Geometry: final body of the model. Coordinates: model frame, mm. A direction names the side the tool comes from. Give positions to 0.01 mm unless a question says otherwise; leave off trailing zeros. Write each loop counter-clockwise with the first axis right and the second up, starting at its lowest first coordinate (ties: lowest second). Pieces come first, ordered by that corner, then holes. Notation, with made-up numbers: (-39, 57.5) - (-21, 57.5) arc R8 ccw to (-21, 67.5) - close; hole circle Ø4 at (20, -12.75). An arc over 180 degrees is marked (long way). Use CSV: the item, a comma, the result in double quotes. Start each with the question number.
(1) Section D-D on z = 5. Output: boundary loops of the cut face in (x, y), and give its area (3 significant figures).
(2) Section C-C on z = 0. Output: boundary loops of the cut face in (x, y), and give its area (3 significant figures).
(3) Line query: probe 1 along Z at (x, y) = (0, -0.5); probe 2 along Y at (x, z) = (-4, -2.25); probe 3 along Z at (x, y) = (18.5, 1.5). Output: solid intervals per line, ascending. Write a range as [from, to].
(4) Draft query along Y for faces 6 (the flat face through (4, -6.5, 2)), 7 (the flat face through (25, 0, 4)), 8 (the flat face through (4, 6.5, 2)), 9 (the flat face through (0.5, -0.1, 7.5)). Return one class per face: released by +Y, released by -Y, zero draft, split by the parting line, or undercut.
(5) Reachability of faces 1 (the flat face through (1, 0, 8)), 2 (the flat face through (19, 0, 3)), 3 (the flat face through (5, 5, 3)), 4 (the flat face through (14, 0, 7.5)), 5 (the cylindrical face through (-6.99, -0.09, -5.67)) from +Z, -Z, +X, -X, +Y, -Y: full face, straight path, thin tool, end or side. Return the list, or none.
(6) Section B-B on x = 18.5. Output: boundary loops of the cut face in (y, z).
(7) Section A-A on y = 2.5. Output: boundary loops of the cut face in (x, z).
(8) First-contact query: pin 1 Ø0.5 at (x, y) = (0.5, 0.5) entering from -Z; pin 2 Ø1.6 at (y, z) = (0, 8.5) entering from -X; pin 3 Ø5 at (x, y) = (4.5, -3) entering from -Z. Flat tips, straight axial feed; report the tip coordinate or a pass-through.
from build123d import *

# Parameters (mm, degrees)
F1_DEPTH = 6.5
F2_T     = -1.5
F3_W     = 2.5
F3_H     = 10
F4_DEPTH = 1.5


with BuildPart() as f1:
    # F0 (on Front) → F1 (new body, symmetric)
    with BuildSketch(Plane.XZ):
        with BuildLine():
            Line((25, 9), (0, 9))
            ThreePointArc((0, 9), (-6.803361, -5.891883), (8.90769, -1.285714))
            ThreePointArc((8.90769, -1.285714), (10.583138, 1.779645), (13.856406, 3))
            Line((13.856406, 3), (25, 3))
            Line((25, 3), (25, 9))
        make_face()
    extrude(amount=F1_DEPTH, both=True)

    # F2
    f2_openings = [f1.faces().sort_by_distance(p)[0] for p in [
        (25, 0, 6),
    ]]
    offset(amount=F2_T, openings=f2_openings)

    # F3 (on face) → F4 (cut)
    with BuildSketch(Plane.XY.offset(9)):
        with Locations((2.25, 0)):
            Rectangle(F3_W, F3_H)
    extrude(amount=-F4_DEPTH, mode=Mode.SUBTRACT)


solid = f1.part
Check values:
1,outline,"(-7.48, -6.5) - (25, -6.5) - (25, -5) - (-5.59, -5) - (-5.59, 5) - (25, 5) - (25, 6.5) - (-7.48, 6.5) - close"
1,area,"116 mm²"
2,outline,"(-9, -6.5) - (9.27, -6.5) - (9.27, 6.5) - (-9, 6.5) - close; hole (-7.5, -5) - (7.67, -5) - (7.67, 5) - (-7.5, 5) - close"
2,area,"85.8 mm²"
3,probe 1,"z = [-9, -7.5], [7.5, 9]"
3,probe 2,"y = [-6.5, -5], [5, 6.5]"
3,probe 3,"z = [3, 4.5], [7.5, 9]"
4,face 6,"released by -Y"
4,face 7,"zero draft"
4,face 8,"released by +Y"
4,face 9,"undercut"
5,face 1,"+Z"
5,face 2,"-Z, +X, +Y, -Y"
5,face 3,"none"
5,face 4,"+X"
5,face 5,"+Y, -Y"
6,outline,"(-6.5, 3) - (6.5, 3) - (6.5, 9) - (-6.5, 9) - close; hole (-5, 4.5) - (5, 4.5) - (5, 7.5) - (-5, 7.5) - close"
7,outline,"(0, 7.5) - (1, 7.5) - (1, 9) - (0, 9) arc R9 ccw (long way) to (8.91, -1.29) arc R5 cw to (13.86, 3) - (25, 3) - (25, 4.5) - (13.86, 4.5) arc R6.5 ccw to (7.42, -1.07) arc R7.5 cw (long way) to start; (3.5, 7.5) - (25, 7.5) - (25, 9) - (3.5, 9) - close"
8,pin 1,"stops at z = -9"
8,pin 2,"stops at x = -4.66"
8,pin 3,"stops at z = -8.77"
